```python
from build123d import *


with BuildPart() as part:
    # 스케치1 → 회전1 (revolve)
    with BuildSketch(Plane(origin=(0, 0, 0), x_dir=(1, 0, 0), z_dir=(0, 1, 0)), mode=Mode.PRIVATE) as revolve_1_sk:
        Polygon((-40, 0), (-40, 25), (-20, 25), (-20, 20), (0, 15), (20, 15), (20, 10), (40, 10), (40, 0), align=None)
    revolve(revolve_1_sk.sketch.rotate(Axis((-49.758874749, 0, 0), (1, 0, 0)), 180), axis=Axis((-49.758874749, 0, 0), (1, 0, 0)))


solid = part.part
```
The listing builds one solid part. Answer for the finished solid, in the listing's coordinates (mm). A direction names the side the tool comes from. Round coordinates to 2 decimals unless told otherwise and drop trailing zeros. Loops run counter-clockwise (first coordinate to the right, second up) from the corner with the lowest first, then second, coordinate; pieces in that order, holes last.
Q1. Section A-A, the plane z = 0 is taken. Determine the outline of the cut face in (x, y), then the cut area to 3 significant figures.
Q2. Given pin 1 Ø1.5 at (y, z) = (-15, 19.5) entering from +X; pin 2 Ø1.5 at (x, z) = (-26, -2.5) entering from -Y; pin 3 Ø2 at (x, z) = (23.5, 8.5) entering from +Y, each flat-ended and moving along its own axis, determine where each tip first touches the part or whether it passes through.
Q3. Find the intervals of material crossed by line 1 (Y direction, x = -33, z = -20); line 2 (X direction, y = -1.5, z = 23.5); line 3 (X direction, y = -8.5, z = -11.5), in increasing order.
Q4. Section D-D, the plane x = 33 is taken. Determine the outline of the cut face in (y, z).
Q5. Section C-C, the plane x = -1 is taken. Determine the outline of the cut face in (y, z).
Q6. Which of the six approach directions +Z, -Z, +X, -X, +Y, -Y give full straight-line access (tool end or side, diameter ignored) to faces 1 (the face through (-40, 0, 0)), 2 (the face through (-20, -17, -11))?
Completed:
1. outline: (-40, -25) - (-20, -25) - (-20, -20) - (0, -15) - (20, -15) - (20, -10) - (40, -10) - (40, 10) - (20, 10) - (20, 15) - (0, 15) - (-20, 20) - (-20, 25) - (-40, 25) - close
1. area: 2,700 mm2
2. pin 1: stops at x = -20
2. pin 2: stops at y = -24.94
2. pin 3: stops at y = 6.61
3. line 1: y = -15 to 15
3. line 2: x = -40 to -20
3. line 3: x = -40 to 20
4. outline: circle Ø20 at (0, 0)
5. outline: circle Ø30.5 at (0, 0)
6. face 1: +Z, -Z, -X, +Y, -Y
6. face 2: +X
